Verification items for the finished model (mm, model axes). A direction names the side the tool comes from. Give positions to 0.01 mm unless a question says otherwise; leave off trailing zeros. Write each loop counter-clockwise with the first axis right and the second up, starting at its lowest first coordinate (ties: lowest second). Pieces come first, ordered by that corner, then holes.
from build123d import *

# Parameters (mm, degrees)
SKETCH2_W                = 101
SKETCH2_H                = 80
BOSS_EXTRUDE1_DEPTH      = 4
BOSS_EXTRUDE2_DEPTH      = 29.4
SKETCH9_R                = 3
BOSS_EXTRUDE3_DEPTH      = 6
M2_5X0_45_TAPPED_HOLE1_D = 2.05


with BuildPart() as part:
    # Sketch2 → Boss-Extrude1 (new body)
    with BuildSketch(Plane(origin=(0, 0, 0), x_dir=(1, 0, 0), z_dir=(0, 1, 0))):
        Rectangle(SKETCH2_W, SKETCH2_H)
    extrude(amount=BOSS_EXTRUDE1_DEPTH)

    # Sketch3 → Boss-Extrude2 (add)
    with BuildSketch(Plane.XZ):
        Polygon((50.5, -40), (-50.5, -40), (-50.5, 40), (-50.5, 44), (-54.5, 44), (-54.5, -44), (54.5, -44), (54.5, 44), (47.5, 44), (47.5, 40), (50.5, 40), align=None)
    extrude(amount=-BOSS_EXTRUDE2_DEPTH)

    # Sketch9 → Boss-Extrude3 (add)
    with BuildSketch(Plane(origin=(0, 4, 0), x_dir=(1, 0, 0), z_dir=(0, 1, 0))):
        with Locations(Location((-46, -22.5, 0), (0, 0, 270))):
            Circle(SKETCH9_R)
        with Locations(Location((-46, 35.5, 0), (0, 0, 270))):
            Circle(SKETCH9_R)
        with Locations(Location((40, 35.5, 0), (0, 0, 270))):
            Circle(SKETCH9_R)
        with Locations(Location((40, -22.5, 0), (0, 0, 270))):
            Circle(SKETCH9_R)
    extrude(amount=BOSS_EXTRUDE3_DEPTH)

    # M2.5x0.45 Tapped Hole1 (through all)
    with Locations(Plane(origin=(0, 10, 0), x_dir=(1, 0, 0), z_dir=(0, 1, 0))):
        with Locations((-46, -22.5), (-46, 35.5), (40, 35.5), (40, -22.5)):
            Hole(M2_5X0_45_TAPPED_HOLE1_D / 2)


solid = part.part
Item 1: Release check for a two-part mould opening along X. For faces 4 (the face through (38.7, 10, 22.5)), 5 (the face through (-1, 0, 1)), 6 (the face through (-54.5, 14, 1)) record: released by +X, released by -X, zero draft, split by the parting line, or undercut.
Answer key:
face 4: undercut
face 5: zero draft
face 6: released by -X
Item 2: Depth check by flat-ended pin: pin 1 (24 mm diameter, centred on x = 4.5, z = -14.5, fed in from +Y); pin 2 (1.2 mm diameter, centred on x = 17.5, y = 3, fed in from +Z); pin 3 (6.5 mm diameter, centred on x = 41, z = 22.5, fed in from +Y). Enter the tip coordinate at first touch or a pass-through.
Answer key:
pin 1: stops at y = 4
pin 2: stops at z = 40
pin 3: stops at y = 10
Item 3: Sectioned sample at C-C on y = 20. Record the cut outline in (x, z), then the cut area to 3 significant figures.
Answer key:
outline: (-54.5, -44) - (54.5, -44) - (54.5, 44) - (47.5, 44) - (47.5, 40) - (50.5, 40) - (50.5, -40) - (-50.5, -40) - (-50.5, 44) - (-54.5, 44) - close
area: 1,120 mm2
Item 4: Set-up check for faces 1 (the face through (50.5, 17, 1)), 2 (the face through (47.5, 14, 42)), 3 (the face through (-46, 10, 24)): record each of +Z, -Z, +X, -X, +Y, -Y from which the full face is reachable in a straight line by a thin tool's end or side.
Answer key:
face 1: +Y
face 2: +Z, +Y, -Y
face 3: +Z, +Y
Item 5: Sectioned sample at D-D on x = 5. Record the cut outline in (y, z), then the cut area to 3 significant figures.
Answer key:
outline: (0, -44) - (29.4, -44) - (29.4, -40) - (4, -40) - (4, 40) - (0, 40) - close
area: 438 mm2
Item 6: Sectioned sample at B-B on z = -9. Record the cut outline in (x, y), then the cut area to 3 significant figures.
Answer key:
outline: (-54.5, 0) - (54.5, 0) - (54.5, 29.4) - (50.5, 29.4) - (50.5, 4) - (-50.5, 4) - (-50.5, 29.4) - (-54.5, 29.4) - close
area: 639 mm2
Item 7: Sectioned sample at A-A on y = 2.75. Record the cut outline in (x, z) (3 decimals).
Answer key:
outline: (-54.5, -44) - (54.5, -44) - (54.5, 44) - (47.5, 44) - (47.5, 40) - (-50.5, 40) - (-50.5, 44) - (-54.5, 44) - close; hole circle Ø2.05 at (-46, -35.5); hole circle Ø2.05 at (-46, 22.5); hole circle Ø2.05 at (40, -35.5); hole circle Ø2.05 at (40, 22.5)
Item 8: Scan lines: line 1 along X through (y, z) = (4.5, -35.5) (3 decimals); line 2 along Z through (x, y) = (40, 3.75) (3 decimals); line 3 along X through (y, z) = (3.5, -35.5) (3 decimals). Record each from-to range of solid material in increasing order.
Answer key:
line 1: x = -54.5 to -50.5, -49 to -47.025, -44.975 to -43, 37 to 38.975, 41.025 to 43, 50.5 to 54.5
line 2: z = -44 to -36.525, -34.475 to 21.475, 23.525 to 40
line 3: x = -54.5 to -47.025, -44.975 to 38.975, 41.025 to 54.5
